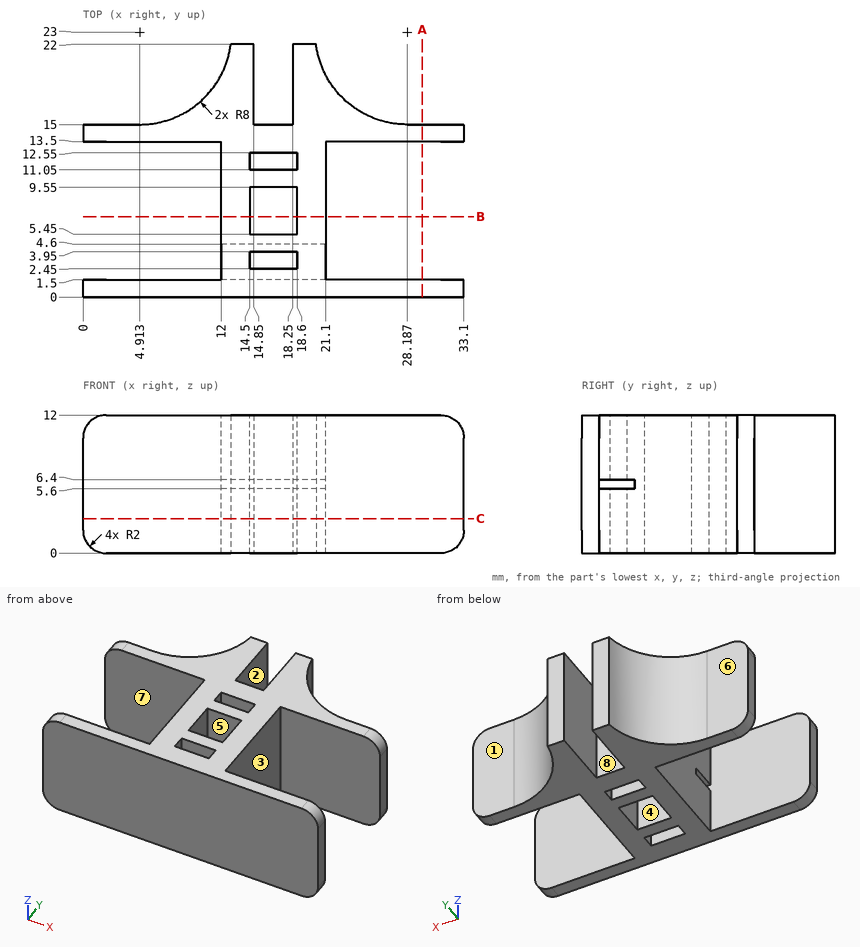
Answer from the drawing. Dimensions are ordinates in mm from the lowest x, y and z of the part. A direction names the side the tool comes from. Coordinates: 2 decimals unless noted, no trailing zeros. Write each loop counter-clockwise with the first axis right and the second up, starting at its lowest first coordinate (ties: lowest second). Pieces come first, ordered by that corner, then holes. Notation, with made-up numbers: (-25.75, -9) - (3.25, -9) arc R22 ccw to (3.25, 7) - close; hole circle Ø4 at (25, -39). An arc over 180 degrees is marked (long way). Answer as CSV lines item,"result".
1. Determine the mould class of the marked faces 1, 2, 3 and 4 for opening direction Y: +Y half, -Y half, draft (parallel to the pull), parting line (faces both ways), or undercut.
Computed values:
face 1,"+Y half"
face 2,"draft"
face 3,"undercut"
face 4,"undercut"
2. Given P1, Ø5.5, axis at x = 2.5, z = 8, coming from the +Y side; P2, Ø3.5, axis at x = 17, z = 4, coming from the -Y side; P3, Ø6, axis at y = 8.5, z = 8.5, coming from the -X side, each flat-ended and moving along its own axis, determine where each tip first touches the part or whether it passes through.
Computed values:
P1,"stops at y = 15.01"
P2,"stops at y = 0"
P3,"stops at x = 12"
3. Find section C-C (z = 3). Give the number of separate pieces and of enclosed holes in the cut face, plus the area to 3 significant figures.
Computed values:
separate pieces,"1"
enclosed holes,"3"
area,"234 mm²"
4. Find section A-A (x = 29.5). Give the vertices of the cut face in (y, z).
Computed values:
outline,"(0, 0) - (1.5, 0) - (1.5, 12) - (0, 12) - close; (13.5, 0) - (15, 0) - (15, 12) - (13.5, 12) - close"
5. A tool of negligible diameter and unlimited length cuts with its end or side. For the marked faces 5, 6, 7 and 8, from which of +Z, -Z, +X, -X, +Y, -Y can it reach the whole face along a straight path? Write none if from no direction.
Computed values:
face 5,"+Z, -Z"
face 6,"+Z, -Z, -X, +Y"
face 7,"+Z, -Z, -X"
face 8,"+Z, -Z, +Y"
6. Find section B-B (y = 7). Give the vertices of the cut face in (x, z), plus the area to 3 significant figures.
Computed values:
outline,"(12, 0) - (14.5, 0) - (14.5, 12) - (12, 12) - close; (18.6, 0) - (21.1, 0) - (21.1, 12) - (18.6, 12) - close"
area,"60.0 mm²"
7. Straight lines are drawn through the part: line 1 (Y direction, x = 18, z = 5.5); line 2 (Y direction, x = 18.5, z = 5.75); line 3 (Y direction, x = 5, z = 5.75). For each, find the intervals that lie inside material, in ascending order. Write a range as [from, to].
Computed values:
line 1,"y = [0, 2.45], [3.95, 5.45], [9.55, 11.05], [12.55, 15]"
line 2,"y = [0, 1.5], [4.6, 5.45], [9.55, 11.05], [12.55, 22]"
line 3,"y = [0, 1.5], [13.5, 15]"
